Could you check a few things on this model? Use its own coordinates, in mm. A direction names the side the tool comes from. Round coordinates to 2 decimals unless told otherwise and drop trailing zeros. Loops run counter-clockwise (first coordinate to the right, second up) from the corner with the lowest first, then second, coordinate; pieces in that order, holes last.
from build123d import *

# Parameters (mm, degrees)
F0_R          = 20
F0_R_2        = 18
F1_DEPTH      = 5
F2_W          = 36
F2_H          = 1.5
F3_DEPTH      = 5
F3_DEPTH_BACK = 95
F4_R          = 20
F5_DEPTH      = 5
F7_DEPTH      = 100.001
F8_R          = 11
F9_DEPTH      = 14.365916731
F10_W         = 25.2537801862
F10_H         = 64.4325390458
F11_DEPTH     = 100


with BuildPart() as f1:
    # F0 (on Front) → F1 (new body)
    with BuildSketch(Plane.XZ):
        Circle(F0_R)
        Circle(F0_R_2, mode=Mode.SUBTRACT)
    extrude(amount=F1_DEPTH)

    # F2 (on Front) → F3 (join, two sides)
    with BuildSketch(Plane.XZ) as f3_sk:
        with Locations((-0.0596572459, -5.75)):
            Rectangle(F2_W, F2_H)
    extrude(amount=F3_DEPTH)
    extrude(f3_sk.sketch, amount=-F3_DEPTH_BACK)

    # F4 (on face) → F5 (join)
    with BuildSketch(Plane(origin=(0, 95, 0), x_dir=(-1, 0, 0), z_dir=(0, 1, 0))):
        Circle(F4_R)
        with BuildLine():
            ThreePointArc((-17.2916164658, -5), (-2.5249657043, 17.8220242451), (18, 0))
            ThreePointArc((18, 0), (17.8220242451, -2.5249657043), (17.2916164658, -5))
            Line((17.2916164658, -5), (18.0596572459, -5))
            Line((18.0596572459, -5), (18.0596572459, -6.5))
            Line((18.0596572459, -6.5), (16.7854103316, -6.5))
            ThreePointArc((16.7854103316, -6.5), (0, -18), (-16.7854103316, -6.5))
            Line((-16.7854103316, -6.5), (-17.9403427541, -6.5))
            Line((-17.9403427541, -6.5), (-17.9403427541, -5))
            Line((-17.9403427541, -5), (-17.2916164658, -5))
        make_face(mode=Mode.SUBTRACT)
    extrude(amount=-F5_DEPTH)

    # F6 (on face) → F7 (cut, through all)
    with BuildSketch(Plane.XZ.offset(5)):
        with BuildLine():
            ThreePointArc((5, -19.364916731), (0, -20), (-5, -19.364916731))
            Line((-5, -19.364916731), (-5, -22.519255057))
            Line((-5, -22.519255057), (5, -22.519255057))
            Line((5, -22.519255057), (5, -19.364916731))
        make_face()
        with BuildLine():
            ThreePointArc((5, -17.2916164658), (0, -18), (-5, -17.2916164658))
            Line((-5, -17.2916164658), (-5, -19.364916731))
            ThreePointArc((-5, -19.364916731), (0, -20), (5, -19.364916731))
            Line((5, -19.364916731), (5, -17.2916164658))
        make_face()
        with BuildLine():
            Line((5, -12.519255057), (-5, -12.519255057))
            Line((-5, -12.519255057), (-5, -17.2916164658))
            ThreePointArc((-5, -17.2916164658), (0, -18), (5, -17.2916164658))
            Line((5, -17.2916164658), (5, -12.519255057))
        make_face()
    extrude(amount=-F7_DEPTH, mode=Mode.SUBTRACT)

    # F8 (on face) → F9 (cut, through all)
    with BuildSketch(Plane.XY.offset(-5)):
        with Locations((0, 12)):
            Circle(F8_R)
        with Locations((0, 45)):
            Circle(F8_R)
        with Locations((0, 78)):
            Circle(F8_R)
    extrude(amount=-F9_DEPTH, mode=Mode.SUBTRACT)

    # F10 (on Front) → F11 (cut, symmetric)
    with BuildSketch(Plane.XZ):
        with Locations((12.6268900931, -0.3540255129)):
            Rectangle(F10_W, F10_H)
    extrude(amount=F11_DEPTH, both=True, mode=Mode.SUBTRACT)


solid = f1.part
Item 1: Will these pins go through, and if not, where does the flat tip stop? pin 1 (1 mm diameter, centred on y = -3, z = -18.5, fed in from +X); pin 2 (6 mm diameter, centred on x = -11, z = -8.5, fed in from +Y); pin 3 (1.5 mm diameter, centred on x = -15.5, z = 2, fed in from -Y); pin 4 (1.5 mm diameter, centred on x = -17.5, y = 68.5, fed in from -Z).
Results list:
pin 1: stops at x = -5
pin 2: stops at y = 95
pin 3: passes through
pin 4: stops at z = -6.5
Item 2: If I drill on line 1 along Z through (x, y) = (-11.5, 59); line 2 along Y through (x, z) = (-12.5, -14), over which ranges is the centre line in solid material (lowest first)?
Results list:
line 1: z = -6.5 to -5
line 2: y = -5 to 0, 90 to 95
Item 3: If we section it at A-A, the plane z = 4.5: Please give me the cut outline in (x, y).
Results list:
outline: (-19.49, -5) - (-17.43, -5) - (-17.43, 0) - (-19.49, 0) - close; (-19.49, 90) - (-17.43, 90) - (-17.43, 95) - (-19.49, 95) - close
Item 4: If we section it at C-C, the plane y = 12: Please give me the cut outline in (x, z).
Results list:
outline: (-18.06, -6.5) - (-11, -6.5) - (-11, -5) - (-18.06, -5) - close
Item 5: If we section it at B-B, the plane x = -9: Count the separate pieces of the cut face and the enclosed holes in it, then the cut area to 3 significant figures.
Results list:
separate pieces: 8
enclosed holes: 0
area: 139 mm2
Item 6: For faces 1 (the flat face through (-18.2, -5, 0.4)), 2 (the flat face through (-5, -3, -18)), which set-ups out of +Z, -Z, +X, -X, +Y, -Y let a thin tool reach every point of the face, with its end or its side?
Results list:
face 1: +Z, -Z, +X, -X, -Y
face 2: -Z, +X, +Y, -Y
Item 7: If we section it at D-D, the plane z = -13: Please give me the cut outline in (x, y), then the cut area to 3 significant figures.
Results list:
outline: (-15.2, -5) - (-12.45, -5) - (-12.45, 0) - (-15.2, 0) - close; (-15.2, 90) - (-12.45, 90) - (-12.45, 95) - (-15.2, 95) - close
area: 27.5 mm2
Item 8: We'd pull the mould along Z, two halves only. Please class faces 3 (the cylindrical face through (-14.25, -2.46, 11)), 4 (the flat face through (-18.2, 0, 1.9)), 5 (the cylindrical face through (-19.887, 92.535, 2.118)): released by +Z, released by -Z, zero draft, split by the parting line, or undercut.
Results list:
face 3: undercut
face 4: zero draft
face 5: split by the parting line
